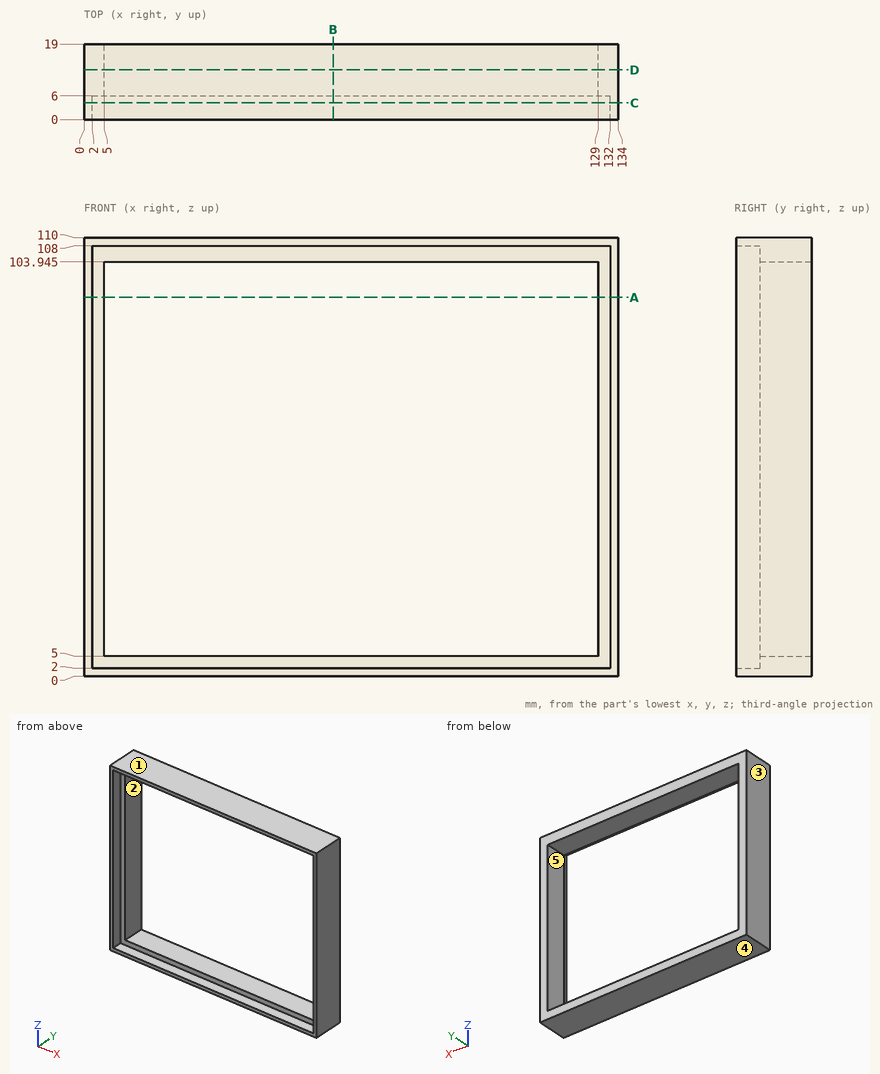
Could you check a few things on this drawing? It's one solid part, dimensions in mm from its lowest x, y, z. A direction names the side the tool comes from. Round coordinates to 2 decimals unless told otherwise and drop trailing zeros. Order: outer loops, then holes, each group sorted by start corner. A loop starts at its lowest first (then second) coordinate and runs counter-clockwise, first axis right, second up. Notation, with made-up numbers: M 18,17 L 53,17 A27 cw 53,56 Z; hole C 36,-38.5 d2. An arc over 180 degrees is marked long. Return JSON: item names as keys, results as strings. Group by question number.
1. If we section it at A-A on z = 95: List the corners of the cut face in (x, y) for me.
2. Please list where these lines run through material, in increasing order: probe 1 along Z at (x, y) = (78, 15) (1 decimal); probe 2 along X at (y, z) = (17, 100); probe 3 along Z at (x, y) = (110, 2.75).
3. On a 3-axis mill with a long thin cutter (end or side, diameter ignored), from which of +Z, -Z, +X, -X, +Y, -Y can I reach the whole of each face in a straight line? I mean the marked faces 1 and 2. Say none if no direction works.
4. If we section it at D-D on y = 12.5: List the corners of the cut face in (x, z) for me (1 decimal).
5. If we section it at B-B on x = 62.5: List the corners of the cut face in (y, z) for me (1 decimal), then the cut area to 3 significant figures.
6. If we section it at C-C on y = 4.25: List the corners of the cut face in (x, z) for me.
7. If we mould it in two halves opening along Z, with no side actions, what happens to the marked faces 3, 4 and 5? For each: pulls with the +Z half, pulls with the -Z half, needs draft (parallel to the pull), parting line crosses it, or undercut.
Reply:
{
 "1": {"outline": "M 0,0 L 2,0 L 2,6 L 5,6 L 5,19 L 0,19 Z; M 129,6 L 132,6 L 132,0 L 134,0 L 134,19 L 129,19 Z"},
 "2": {"probe 1": "0 to 5, 103.9 to 110", "probe 2": "0 to 5, 129 to 134", "probe 3": "0 to 2, 108 to 110"},
 "3": {"face 1": "+Z, +X, -X, +Y, -Y", "face 2": "+Y, -Y"},
 "4": {"outline": "M 0,0 L 134,0 L 134,110 L 0,110 Z; hole M 5,5 L 129,5 L 129,103.9 L 5,103.9 Z"},
 "5": {"outline": "M 0,0 L 19,0 L 19,5 L 6,5 L 6,2 L 0,2 Z; M 0,108 L 6,108 L 6,103.9 L 19,103.9 L 19,110 L 0,110 Z", "area": "168 mm^2"},
 "6": {"outline": "M 0,0 L 134,0 L 134,110 L 0,110 Z; hole M 2,2 L 132,2 L 132,108 L 2,108 Z"},
 "7": {"face 3": "needs draft", "face 4": "pulls with the -Z half", "face 5": "undercut"}
}
